```python
from build123d import *

# Parameters (mm, degrees)
F0_W     = 100
F0_H     = 100
F1_DEPTH = 10
F3_DEPTH = 8


with BuildPart() as f1:
    # F0 (on Top) → F1 (new body)
    with BuildSketch(Plane.XY):
        Rectangle(F0_W, F0_H)
    extrude(amount=F1_DEPTH)

    # F2 (on face) → F3 (join)
    with BuildSketch(Plane.XY.offset(10)):
        with BuildLine():
            ThreePointArc((-15.098755, 36.308361), (-20.017806, 35.458787), (-15.034038, 35.743209))
            ThreePointArc((-15.034038, 35.743209), (-15.05027, 36.027632), (-15.098755, 36.308361))
        make_face()
        with BuildLine():
            ThreePointArc((30.956892, -27.842858), (30.569075, -26.505442), (29.525946, -25.582964))
            ThreePointArc((29.525946, -25.582964), (26.344709, -29.180275), (30.956892, -27.842858))
        make_face()
        with BuildLine():
            ThreePointArc((42.075047, -4.339951), (41.160451, -2.40695), (39.085853, -1.888281))
            Line((39.085853, -1.888281), (39.575047, -4.339951))
            Line((39.575047, -4.339951), (38.505993, -6.599846))
            ThreePointArc((38.505993, -6.599846), (40.912463, -6.452134), (42.075047, -4.339951))
        make_face()
        with BuildLine():
            Line((39.575047, -4.339951), (39.085853, -1.888281))
            ThreePointArc((39.085853, -1.888281), (37.093767, -4.034577), (38.505993, -6.599846))
            Line((38.505993, -6.599846), (39.575047, -4.339951))
        make_face()
        with BuildLine():
            ThreePointArc((37.378786, 19.196088), (35.838191, 21.504668), (33.115153, 20.967979))
            Line((33.115153, 20.967979), (34.878786, 19.196088))
            Line((34.878786, 19.196088), (35.36798, 16.744417))
            ThreePointArc((35.36798, 16.744417), (36.811787, 17.610683), (37.378786, 19.196088))
        make_face()
        with BuildLine():
            Line((34.878786, 19.196088), (33.115153, 20.967979))
            ThreePointArc((33.115153, 20.967979), (32.67296, 18.019511), (35.36798, 16.744417))
            Line((35.36798, 16.744417), (34.878786, 19.196088))
        make_face()
        with BuildLine():
            ThreePointArc((21.858815, 34.78873), (19.675335, 37.268612), (16.938963, 35.416677))
            Line((16.938963, 35.416677), (19.358815, 34.78873))
            Line((19.358815, 34.78873), (21.122448, 33.016839))
            ThreePointArc((21.122448, 33.016839), (21.667395, 33.829325), (21.858815, 34.78873))
        make_face()
        with BuildLine():
            Line((19.358815, 34.78873), (16.938963, 35.416677))
            ThreePointArc((16.938963, 35.416677), (18.114845, 32.620197), (21.122448, 33.016839))
            Line((21.122448, 33.016839), (19.358815, 34.78873))
        make_face()
        with BuildLine():
            ThreePointArc((2.5, 39.812303), (-0.284423, 42.296071), (-2.435283, 39.247151))
            Line((-2.435283, 39.247151), (0, 39.812303))
            Line((0, 39.812303), (2.419852, 39.184357))
            ThreePointArc((2.419852, 39.184357), (2.479882, 39.495783), (2.5, 39.812303))
        make_face()
        with BuildLine():
            Line((0, 39.812303), (-2.435283, 39.247151))
            ThreePointArc((-2.435283, 39.247151), (-0.032331, 37.312512), (2.419852, 39.184357))
            Line((2.419852, 39.184357), (0, 39.812303))
        make_face()
    extrude(amount=F3_DEPTH)


solid = f1.part
```
Work out the finished part from the listing and answer in its coordinate system (mm). Round coordinates to 2 decimals unless told otherwise and drop trailing zeros. Loops run counter-clockwise (first coordinate to the right, second up) from the corner with the lowest first, then second, coordinate; pieces in that order, holes last.
(1) Each of these flat-tipped pins is pushed along its axis until it touches: P1, Ø1, axis at x = 15, y = 22.5, coming from the -Z side; P2, Ø1, axis at x = -30.5, y = 14, coming from the +Z side. Where does it stop, or does it pass through?
Computed values:
P1: stops at z = 0
P2: stops at z = 10
(2) The part is cut by section C-C, the plane y = -40.5. Give the vertices of the cut face in (x, z), and give its area (3 significant figures).
Computed values:
outline: (-50, 0) - (50, 0) - (50, 10) - (-50, 10) - close
area: 1,000 mm2
(3) The part is cut by section A-A, the plane z = 13. Give the vertices of the cut face in (x, y), and give its area (3 significant figures).
Computed values:
outline: (-15.1, 36.31) arc R2.5 ccw (long way) to (-15.03, 35.74) arc R2.5 ccw to start; (2.42, 39.18) arc R2.5 ccw to (2.5, 39.81) arc R2.5 ccw (long way) to start; circle Ø5 at (19.36, 34.79); circle Ø5 at (28.46, -27.84); circle Ø5 at (34.88, 19.2); (38.51, -6.6) arc R2.5 ccw to (42.08, -4.34) arc R2.5 ccw to (39.09, -1.89) arc R2.5 ccw to start
area: 118 mm2
(4) The part is cut by section B-B, the plane x = 0. Give the vertices of the cut face in (y, z), and give its area (3 significant figures).
Computed values:
outline: (-50, 0) - (50, 0) - (50, 10) - (42.31, 10) - (42.31, 18) - (37.31, 18) - (37.31, 10) - (-50, 10) - close
area: 1,040 mm2
(5) Find the intervals of material crossed by L1, parallel to Z at x = -32, y = 32; L2, parallel to X at y = -26, z = 11.75, in increasing order.
Computed values:
L1: z = 0 to 10
L2: x = 26.77 to 30.15
